Build history of the part. All positions in model axes, mm. A direction names the side the tool comes from. Round coordinates to 2 decimals unless told otherwise and drop trailing zeros. Loops run counter-clockwise (first coordinate to the right, second up) from the corner with the lowest first, then second, coordinate; pieces in that order, holes last. Notation, with made-up numbers: (0.5, -22.5) - (5.5, -22.5) arc R28 ccw to (5.5, 7.5) - close; hole circle Ø8 at (19, 80.5). An arc over 180 degrees is marked (long way). Answer as CSV lines item,"result". Start each with the question number.
Autodesk Inventor part; units mm, degrees
ref_plane "YZ Plane" through (0, 0, 0) normal (1, 0, 0) x (0, 1, 0)
ref_plane "XZ Plane" through (0, 0, 0) normal (0, 1, 0) x (-1, 0, 0)
ref_plane "XY Plane" through (0, 0, 0) normal (0, 0, 1) x (1, 0, 0)
sketch "Sketch1" plane through (0, 0, 0) normal (0, 0, 1) x (1, 0, 0)
  line L0 (5.6515, 0) -> (36.6485, 0)
  line L1 (42.3, 5.6515) -> (42.3, 36.6485)
  line L2 (36.6485, 42.3) -> (5.6515, 42.3)
  line L3 (0, 36.6485) -> (0, 5.6515)
  line L4 (0, 36.6485) -> (5.6515, 42.3)
  line L5 (36.6485, 42.3) -> (42.3, 36.6485)
  line L6 (42.3, 5.6515) -> (36.6485, 0)
  line L7 (5.6515, 0) -> (0, 5.6515)
  line L8 (21.15, 42.3) -> (21.15, 0) construction
  line L9 (0, 21.9578) -> (42.3, 21.9578) construction
  point P0 (0, 0)
  point P1 (42.3, 42.3)
  point P2 (42.3, 0)
  point P3 (0, 42.3)
  dimension "d0" = 42.3
  dimension "d1" = 42.3
  dimension "d2" = 5.6515
  dimension "d3" = 5.6515
  dimension "d4" = 5.6515
  dimension "d5" = 5.6515
  dimension "d6" = 5.6515
  dimension "d7" = 5.6515
  dimension "d8" = 5.6515
  dimension "d9" = 5.6515
  dimension "d10" = 30.997
extrude "Extrusion1" add sketch "Sketch1" along normal blind 33.02
sketch "Sketch2" plane through (0, 0, 33.02) normal (0, 0, 1) x (1, 0, 0)
  line L0 (5.6515, 42.3) -> (36.6485, 42.3)
  line L1 (0, 5.6515) -> (0, 36.6485)
  line L2 (36.6485, 0) -> (5.6515, 0)
  line L3 (42.3, 36.6485) -> (42.3, 5.6515)
  line L4 (21.15, 42.3) -> (21.15, 0) construction
  line L5 (0, 21.15) -> (42.3, 21.15) construction
  circle A0 centre (21.15, 21.15) radius 11
  point P0 (0, 0)
  dimension "d13" = 22
extrude "Extrusion2" add sketch "Sketch2" along normal blind 2
sketch "Sketch3" plane through (21.15, 21.15, 35.02) normal (0, 0, 1) x (1, 0, 0)
  circle A0 centre (0, 0) radius 11
  arc A1 (0.6085, 2.4399) -> (2.2645, -1.0932) centre (0, 0) ccw
  line L0 (0.6085, 2.4399) -> (2.2645, -1.0932)
  line L1 (1.4365, 0.6733) -> (-2.2769, -1.0672) construction
  point P0 (-21.15, -21.15)
  dimension "d16" = 5.0292
  dimension "d34" = 3.9019
  dimension "d36" = 1.951
  dimension "d37" = 4.1011
extrude "Extrusion3" add sketch "Sketch3" along normal blind 16.002 contours L0 A1
sketch "Sketch4" plane through (0, 0, 33.02) normal (0, 0, 1) x (1, 0, 0)
  line L0 (0, 36.6485) -> (5.6515, 42.3)
  line L1 (5.6515, 0) -> (0, 5.6515)
  line L2 (42.3, 5.6515) -> (36.6485, 0)
  line L3 (36.6485, 42.3) -> (42.3, 36.6485)
  line L4 (2.8258, 39.4742) -> (39.4742, 2.8258) construction
  line L5 (39.4742, 39.4742) -> (2.8257, 2.8258) construction
  point P0 (0, 0)
  point P1 (5.65, 36.65)
  point P2 (36.65, 36.65)
  point P3 (5.65, 5.65)
  point P4 (36.65, 5.65)
  dimension "d20" = 31
  dimension "d21" = 31
  dimension "d22" = 31
  dimension "d23" = 31
hole "Hole1" at (5.65, 36.65, 33.02) at (36.65, 36.65, 33.02) at (5.65, 5.65, 33.02) at (36.65, 5.65, 33.02) direction (0, 0, -1) diameter 4 end through all
equation "\"d36\" = 0.5 * d34"
properties part number "stepper42BYGH007_RB01" material "Aluminum-6061"
Q1. Tool access for faces 5 (the flat face through (0, 21, 16)), 6 (the cylindrical face through (18.91, 20.01, 42.91)): list every direction of +Z, -Z, +X, -X, +Y, -Y with a clear straight run to the whole face (end or side of a thin tool).
Q2. Band-saw the part on C-C, the plane y = 21.15. List the corners of the cut face in (x, z).
Q3. Pin check, flat tips, straight feed: pin 1 Ø3.5 at (x, y) = (5.65, 5.65) entering from -Z; pin 2 Ø10 at (x, y) = (31.5, 29.5) entering from +Z; pin 3 Ø5 at (x, y) = (35, 17.5) entering from +Z. Stop position of each tip, or through.
Q4. Band-saw the part on D-D, the plane x = 25. List the corners of the cut face in (y, z).
Q5. Wall check: probe 1 along X at (y, z) = (36.65, 16.5); probe 2 along Y at (x, z) = (5.5, 9.5). Give the ranges that are in metal, low to high. Write a range as [from, to].
Q6. Two-plate mould, pull along X, no slides. Class faces 1 (the cylindrical face through (37.416, 3.803, 16.279)), 2 (the flat face through (21, 21, 0)), 3 (the flat face through (22.575, 21.848, 42.909)), 4 (the cylindrical face through (6.416, 34.803, 16.279)): released by +X, released by -X, zero draft, split by the parting line, or undercut.
Q7. Band-saw the part on B-B, the plane y = 35.5. List the corners of the cut face in (x, z), then the cut area to 3 significant figures.
Q8. Band-saw the part on A-A, the plane z = 11.5. List the corners of the cut face in (x, y).
Reported:
1,face 5,"+Z, -Z, -X, +Y, -Y"
1,face 6,"+Z"
2,outline,"(0, 0) - (42.3, 0) - (42.3, 33.02) - (32.15, 33.02) - (32.15, 35.02) - (22.9, 35.02) - (22.9, 51.02) - (18.64, 51.02) - (18.64, 35.02) - (10.15, 35.02) - (10.15, 33.02) - (0, 33.02) - close"
3,pin 1,"passes through"
3,pin 2,"stops at z = 35.02"
3,pin 3,"stops at z = 33.02"
4,outline,"(0, 0) - (42.3, 0) - (42.3, 33.02) - (31.45, 33.02) - (31.45, 35.02) - (10.85, 35.02) - (10.85, 33.02) - (0, 33.02) - close"
5,probe 1,"x = [0, 3.65], [7.65, 34.65], [38.65, 42.3]"
5,probe 2,"y = [0.15, 3.66], [7.64, 34.66], [38.64, 42.15]"
6,face 1,"undercut"
6,face 2,"zero draft"
6,face 3,"released by +X"
6,face 4,"undercut"
7,outline,"(0, 0) - (4.01, 0) - (4.01, 33.02) - (0, 33.02) - close; (7.29, 0) - (35.01, 0) - (35.01, 33.02) - (7.29, 33.02) - close; (38.29, 0) - (42.3, 0) - (42.3, 33.02) - (38.29, 33.02) - close"
7,area,"1,180 mm2"
8,outline,"(0, 5.65) - (5.65, 0) - (36.65, 0) - (42.3, 5.65) - (42.3, 36.65) - (36.65, 42.3) - (5.65, 42.3) - (0, 36.65) - close; hole circle Ø4 at (5.65, 5.65); hole circle Ø4 at (5.65, 36.65); hole circle Ø4 at (36.65, 5.65); hole circle Ø4 at (36.65, 36.65)"
